Here's how the part is built. I have some questions about the finished solid (model axes, mm). A direction names the side the tool comes from. Round coordinates to 2 decimals unless told otherwise and drop trailing zeros. Write each loop counter-clockwise with the first axis right and the second up, starting at its lowest first coordinate (ties: lowest second). Pieces come first, ordered by that corner, then holes. Notation, with made-up numbers: M 26.25,33.25 L 60.25,33.25 A8 ccw 60.25,45.25 Z; hole C 10.5,19.5 d2. An arc over 180 degrees is marked long. Write item = value, one per line. Start each with the question number.
(1) I want a section at A-A (z = 7.75). List the corners of the cut face in (x, y) for me.
(2) On a 3-axis mill with a long thin cutter (end or side, diameter ignored), from which of +Z, -Z, +X, -X, +Y, -Y can I reach the whole of each face in a straight line? I mean faces 5 (the cylindrical face through (7.475, 39.201, 5.07)), 6 (the flat face through (0, 1, 0)), 7 (the flat face through (-7, 1, 5)). Say none if no direction works.
(3) I need wall thicknesses on line 1 along Y through (x, z) = (0, 7.25); line 2 along Y through (x, z) = (3, 5.75); line 3 along Y through (x, z) = (-3.25, 5.75). Which ranges of each line are inside material? Lowest first, please.
(4) If we mould it in two halves opening along X, with no side actions, what happens to faces 1 (the cylindrical face through (2.42, 52.28, 4.93)), 2 (the flat face through (7, -1, 5)), 3 (the cylindrical face through (-7.475, -39.201, 5.07)), 4 (the cylindrical face through (-1.084, -53.366, 5.07))? For each: released by +X, released by -X, zero draft, split by the parting line, or undercut.
(5) Will these pins go through, and if not, where does the flat tip stop? pin 1 Ø4 at (x, z) = (7.5, 1.5) entering from +Y; pin 2 Ø1 at (x, z) = (-7.5, 1) entering from -Y; pin 3 Ø5 at (y, z) = (-13.5, 5.5) entering from -X; pin 4 Ø8 at (x, y) = (0, -48.49) entering from -Z.
(6) I want a section at B-B (x = -3.25). List the corners of the cut face in (y, z) for me.
(7) I want a section at C-C (y = 1.5). List the corners of the cut face in (x, z) for me, and give its area (3 significant figures).
```python
from build123d import *

# Parameters (mm, degrees)
ESQUISSE1_R                 = 4.502635458
BOSS_EXTRU_1_DEPTH          = 10
TROU_TARAUD_M22_D           = 1.6
TROU_TARAUD_M22_CSINK_D     = 2.05
TROU_TARAUD_M22_CSINK_ANGLE = 90
CONG_1_R                    = 10
ESQUISSE9_R                 = 5
ENL_V_MAT_EXTRU_1_DEPTH     = 10


with BuildPart() as part:
    # Esquisse1 → Boss.-Extru.1 (new body)
    with BuildSketch(Plane.XY):
        with BuildLine():
            Line((-7, 40), (-7, -40))
            ThreePointArc((-7, -40), (0, -59.485281374), (7, -40))
            Line((7, -40), (7, 40))
            ThreePointArc((7, 40), (0, 59.485281374), (-7, 40))
        make_face()
        with Locations((0, 48.485281374)):
            Circle(ESQUISSE1_R, mode=Mode.SUBTRACT)
    extrude(amount=BOSS_EXTRU_1_DEPTH)

    # Trou taraudé M22 (through all)
    with Locations(Plane.XY.offset(10)):
        with Locations((-8, 48.485281374), (0, 56.485281374), (8, 48.485281374), (0, 40.485281374)):
            CounterSinkHole(TROU_TARAUD_M22_D / 2, TROU_TARAUD_M22_CSINK_D / 2, counter_sink_angle=TROU_TARAUD_M22_CSINK_ANGLE)

    # Congé1
    cong_1_edges = [part.edges().sort_by_distance(p)[0] for p in [
        (7, 40, 5),
        (7, -40, 5),
        (-7, -40, 5),
        (-7, 40, 5),
    ]]
    fillet(cong_1_edges, radius=CONG_1_R)

    # Esquisse9 → Enlèv. mat.-Extru.1 (cut)
    with BuildSketch(Plane.XY.offset(10)):
        with Locations((0, -48.485281374)):
            Circle(ESQUISSE9_R)
    extrude(amount=-ENL_V_MAT_EXTRU_1_DEPTH, mode=Mode.SUBTRACT)


solid = part.part
```
Returned:
q1.outline = M -8.9,-42.03 A11 ccw long 8.9,-42.03 A10 cw 7,-36.16 L 7,36.16 A10 cw 8.9,42.03 A11 ccw long -8.9,42.03 A10 cw -7,36.16 L -7,-36.16 A10 cw Z; hole C -8,48.49 d1.6; hole C 0,-48.49 d10; hole C 0,48.49 d9.01; hole C 0,40.49 d1.6; hole C 0,56.49 d1.6; hole C 8,48.49 d1.6
q2.face_5 = +Z, -Z, +X
q2.face_6 = -Z, +X, -X, +Y, -Y
q2.face_7 = +Z, -Z, -X
q3.line_1 = -59.49 to -53.49, -43.49 to 39.69, 41.29 to 43.98, 52.99 to 55.69, 57.29 to 59.49
q3.line_2 = -59.07 to -52.49, -44.49 to 45.13, 51.84 to 59.07
q3.line_3 = -58.99 to -52.28, -44.69 to 45.37, 51.6 to 58.99
q4.face_1 = undercut
q4.face_2 = released by +X
q4.face_3 = released by -X
q4.face_4 = undercut
q5.pin_1 = 58.01
q5.pin_2 = -56.97
q5.pin_3 = -7
q5.pin_4 = through
q6.outline = M -58.99,0 L -52.28,0 L -52.28,10 L -58.99,10 Z; M -44.69,0 L 45.37,0 L 45.37,10 L -44.69,10 Z; M 51.6,0 L 58.99,0 L 58.99,10 L 51.6,10 Z
q7.outline = M -7,0 L 7,0 L 7,10 L -7,10 Z
q7.area = 140 mm²
